from build123d import *

# Parameters (mm, degrees)
EXTRUDE_4_DEPTH     = 10
EXTRUDE_3_DEPTH     = 1.5
CUT_EXTRUDE_2_REACH = 57.745
SKETCH_7_W          = 14
SKETCH_7_H          = 5
SKETCH_8_R          = 2.076581153
SKETCH_8_R_2        = 0.576581153
EXTRUDE_5_DEPTH     = 2.75
EXTRUDE_4_2_DEPTH   = 8.5


with BuildPart() as part:
    # 草图3 → Extrude 4 (new body)
    with BuildSketch(Plane(origin=(0, 0, 0), x_dir=(1, 0, 0), z_dir=(0, 1, 0))):
        with BuildLine():
            Line((50.567091694, 22.728702057), (1.78119206, 22.728702057))
            ThreePointArc((1.78119206, 22.728702057), (-0.678586397, 21.70982846), (-1.697459995, 19.250050003))
            Line((-1.697459995, 19.250050003), (-1.697459995, 1.905652309))
            ThreePointArc((-1.697459995, 1.905652309), (-0.678586397, -0.554126149), (1.78119206, -1.572999746))
            Line((1.78119206, -1.572999746), (50.567091694, -1.572999746))
            ThreePointArc((50.567091694, -1.572999746), (53.027823293, -0.553731345), (54.047091694, 1.907000254))
            Line((54.047091694, 1.907000254), (54.047091694, 19.248702057))
            ThreePointArc((54.047091694, 19.248702057), (53.027823293, 21.709433656), (50.567091694, 22.728702057))
        make_face()
        with BuildLine():
            Line((50.567091694, 21.228702057), (1.78119206, 21.228702057))
            ThreePointArc((1.78119206, 21.228702057), (0.382073774, 20.649168288), (-0.197459995, 19.250050003))
            Line((-0.197459995, 19.250050003), (-0.197459995, 1.905652309))
            ThreePointArc((-0.197459995, 1.905652309), (0.382073774, 0.506534023), (1.78119206, -0.072999746))
            Line((1.78119206, -0.072999746), (50.567091694, -0.072999746))
            ThreePointArc((50.567091694, -0.072999746), (51.967163121, 0.506928827), (52.547091694, 1.907000254))
            Line((52.547091694, 1.907000254), (52.547091694, 19.248702057))
            ThreePointArc((52.547091694, 19.248702057), (51.967163121, 20.648773484), (50.567091694, 21.228702057))
        make_face(mode=Mode.SUBTRACT)
    extrude(amount=EXTRUDE_4_DEPTH)

    # 草图3<5> → 凸台-拉伸3 (add)
    with BuildSketch(Plane(origin=(0, 0, 0), x_dir=(1, 0, 0), z_dir=(0, 1, 0))):
        with BuildLine():
            Line((50.567091694, 21.228702057), (1.78119206, 21.228702057))
            ThreePointArc((1.78119206, 21.228702057), (0.382073774, 20.649168288), (-0.197459995, 19.250050003))
            Line((-0.197459995, 19.250050003), (-0.197459995, 1.905652309))
            ThreePointArc((-0.197459995, 1.905652309), (0.382073774, 0.506534023), (1.78119206, -0.072999746))
            Line((1.78119206, -0.072999746), (50.567091694, -0.072999746))
            ThreePointArc((50.567091694, -0.072999746), (51.967163121, 0.506928827), (52.547091694, 1.907000254))
            Line((52.547091694, 1.907000254), (52.547091694, 19.248702057))
            ThreePointArc((52.547091694, 19.248702057), (51.967163121, 20.648773484), (50.567091694, 21.228702057))
        make_face()
    extrude(amount=EXTRUDE_3_DEPTH)

    # 草图7 → 切除-拉伸2 (cut, up to next)
    with BuildSketch(Plane(origin=(54.047091694, 0, 0), x_dir=(0, 0, -1), z_dir=(1, 0, 0)), mode=Mode.PRIVATE) as cut_extrude_2_sk1:
        with Locations((10.577851156, 5)):
            Rectangle(SKETCH_7_W, SKETCH_7_H)
    cut_extrude_2_tool1 = extrude(cut_extrude_2_sk1.sketch, amount=-CUT_EXTRUDE_2_REACH, mode=Mode.PRIVATE) & part.part
    add(cut_extrude_2_tool1.solids().sort_by_distance((54.047092, 5, -10.577851))[0], mode=Mode.SUBTRACT)

    # 草图8 → 拉伸-薄壁5 (add)
    with BuildSketch(Plane(origin=(0, 1.5, 0), x_dir=(1, 0, 0), z_dir=(0, 1, 0))):
        with Locations((44.069088138, 1.90500381)):
            Circle(SKETCH_8_R)
        with Locations((44.069088138, 1.90500381)):
            Circle(SKETCH_8_R_2, mode=Mode.SUBTRACT)
        with Locations((44.069088138, 19.250698501)):
            Circle(SKETCH_8_R)
        with Locations((44.069088138, 19.250698501)):
            Circle(SKETCH_8_R_2, mode=Mode.SUBTRACT)
        with Locations((1.780543561, 19.250698501)):
            Circle(SKETCH_8_R)
        with Locations((1.780543561, 19.250698501)):
            Circle(SKETCH_8_R_2, mode=Mode.SUBTRACT)
        with Locations((1.780543561, 1.90500381)):
            Circle(SKETCH_8_R)
        with Locations((1.780543561, 1.90500381)):
            Circle(SKETCH_8_R_2, mode=Mode.SUBTRACT)
    extrude(amount=EXTRUDE_5_DEPTH)

    # 草图9 → Extrude 4 2 (add)
    with BuildSketch(Plane(origin=(0, 1.5, 0), x_dir=(1, 0, 0), z_dir=(0, 1, 0))):
        with BuildLine():
            Line((44.70129951, -0.072999746), (50.567091694, -0.072999746))
            ThreePointArc((50.567091694, -0.072999746), (51.967163121, 0.506928827), (52.547091694, 1.907000254))
            Line((52.547091694, 1.907000254), (46.145668332, 1.907000254))
            ThreePointArc((46.145668332, 1.907000254), (45.746731704, 0.681197718), (44.70129951, -0.072999746))
        make_face()
        with BuildLine():
            Line((44.70129951, 21.228702057), (50.567091694, 21.228702057))
            ThreePointArc((50.567091694, 21.228702057), (51.967163121, 20.648773484), (52.547091694, 19.248702057))
            Line((52.547091694, 19.248702057), (46.145668332, 19.248702057))
            ThreePointArc((46.145668332, 19.248702057), (45.746731704, 20.474504593), (44.70129951, 21.228702057))
        make_face()
    extrude(amount=EXTRUDE_4_2_DEPTH)


solid = part.part
Read the model definition and answer for the solid it produces. Units are mm, in the model's axes. A direction names the side the tool comes from. Give positions to 0.01 mm unless a question says otherwise; leave off trailing zeros. Write each loop counter-clockwise with the first axis right and the second up, starting at its lowest first coordinate (ties: lowest second). Pieces come first, ordered by that corner, then holes. Notation, with made-up numbers: (-35, 47.5) - (13, 47.5) arc R11 cw to (13, 66.5) - close; hole circle Ø7 at (16, 82.25). An arc over 180 degrees is marked (long way). Answer in a Markdown table with one row per item. Add a question column.
Item 1: Section A-A, the plane z = -8.5 is taken. Write down the section's boundary in (x, y), and give its area (3 significant figures).
Item 2: Find the intervals of material crossed by L1, parallel to X at y = 6.5, z = -3; L2, parallel to Z at x = 24, y = 3.75; L3, parallel to X at y = 3, z = -19.5, in increasing order.
Item 3: Section B-B, the plane x = 37 is taken. Write down the section's boundary in (y, z), and give its area (3 significant figures).
Item 4: A tool of negligible diameter and unlimited length cuts with its end or side. For faces 1 (the face through (26, 1.5, -11)), 2 (the face through (27, 5, -22.729)), 3 (the face through (53, 2.5, -10)), from which of +Z, -Z, +X, -X, +Y, -Y can it reach the whole face along a straight path? Write none if from no direction.
Item 5: Section C-C, the plane x = 51.5 is taken. Write down the section's boundary in (y, z), and give its area (3 significant figures).
Item 6: Determine the mould class of faces 4 (the face through (26, 0, -11)), 5 (the face through (49, 6, -1.907)), 6 (the face through (23, 6, 0.073)), 7 (the face through (53, 4.93, 0.58)) for opening direction Z: pulls with the +Z half, pulls with the -Z half, needs draft (parallel to the pull), parting line crosses it, or undercut.
Item 7: Flat-ended cylindrical pins translate along their axes: P1, Ø1.2, axis at x = 44.5, z = -20, coming from the +Y side; P2, Ø1.6, axis at x = 53, y = 4, coming from the +Z side; P3, Ø4, axis at x = 28.5, z = -13.5, coming from the +Y side. Find the tip coordinate at first contact, or state that the pin passes through.
Item 8: Section D-D, the plane x = 44 is taken. Write down the section's boundary in (y, z).
Recorded:
| question | item | result |
|---|---|---|
| 1 | outline | (-1.7, 0) - (54.05, 0) - (54.05, 2.5) - (52.55, 2.5) - (52.55, 1.5) - (-0.2, 1.5) - (-0.2, 10) - (-1.7, 10) - close; (52.55, 7.5) - (54.05, 7.5) - (54.05, 10) - (52.55, 10) - close |
| 1 | area | 102 mm2 |
| 2 | L1 | x = -1.7 to -0.2, 52.55 to 54.05 |
| 2 | L2 | z = -22.73 to -21.23, 0.07 to 1.57 |
| 2 | L3 | x = -1.69 to 1.26, 2.3 to 3.84, 42.01 to 43.55, 44.59 to 54.04 |
| 3 | outline | (0, -22.73) - (10, -22.73) - (10, -21.23) - (1.5, -21.23) - (1.5, 0.07) - (10, 0.07) - (10, 1.57) - (0, 1.57) - close |
| 3 | area | 62.0 mm2 |
| 4 | face 1 | +Y |
| 4 | face 2 | -Z, +X, -X, +Y, -Y |
| 4 | face 3 | +X |
| 5 | outline | (0, -22.6) - (10, -22.6) - (10, -19.25) - (1.5, -19.25) - (1.5, -1.91) - (10, -1.91) - (10, 1.45) - (0, 1.45) - close |
| 5 | area | 93.1 mm2 |
| 6 | face 4 | needs draft |
| 6 | face 5 | undercut |
| 6 | face 6 | undercut |
| 6 | face 7 | pulls with the +Z half |
| 7 | P1 | stops at y = 4.25 |
| 7 | P2 | stops at z = 1.17 |
| 7 | P3 | stops at y = 1.5 |
| 8 | outline | (0, -22.73) - (10, -22.73) - (10, -21.23) - (4.25, -21.23) - (4.25, -19.82) - (1.5, -19.82) - (1.5, -18.68) - (4.25, -18.68) - (4.25, -17.18) - (1.5, -17.18) - (1.5, -3.98) - (4.25, -3.98) - (4.25, -2.48) - (1.5, -2.48) - (1.5, -1.33) - (4.25, -1.33) - (4.25, 0.07) - (10, 0.07) - (10, 1.57) - (0, 1.57) - close |
